Drawing for the job (mm, zero at the part's lowest x, y, z). A direction names the side the tool comes from. Round coordinates to 2 decimals unless told otherwise and drop trailing zeros. Loops run counter-clockwise (first coordinate to the right, second up) from the corner with the lowest first, then second, coordinate; pieces in that order, holes last. Notation, with made-up numbers: M 88,64 L 92,64 A23 ccw 92,73 Z; hole C 82,39.25 d1. An arc over 180 degrees is marked long. Answer in a Markdown table with one row per item.
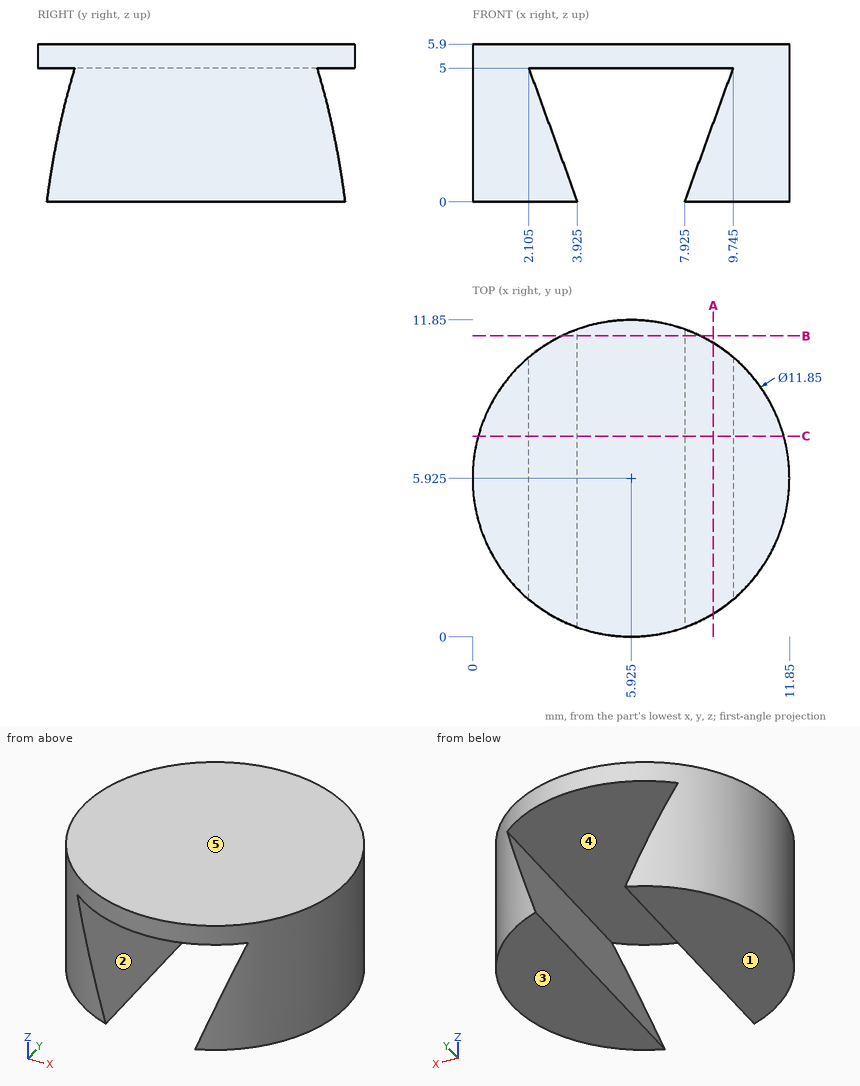
1. Saw through at A-A (x = 9). Write the cut outline in (y, z), and give its area (3 significant figures).
Verdict:
| item | result |
|---|---|
| outline | M 0.86,0 L 10.99,0 L 10.99,2.95 L 0.86,2.95 Z; M 0.86,5 L 10.99,5 L 10.99,5.9 L 0.86,5.9 Z |
| area | 39.0 mm² |
2. Mould opens along Z. For the marked faces 3, 4 and 5 say: +Z half, -Z half, draft (parallel to the pull), parting line (faces both ways), or undercut.
Verdict:
| item | result |
|---|---|
| face 3 | -Z half |
| face 4 | undercut |
| face 5 | +Z half |
3. Tool access for the marked faces 1 and 2: list every direction of +Z, -Z, +X, -X, +Y, -Y with a clear straight run to the whole face (end or side of a thin tool).
Verdict:
| item | result |
|---|---|
| face 1 | -Z, +X, -X, +Y, -Y |
| face 2 | +Y, -Y |
4. Pin check, flat tips, straight feed: pin 1 (4 mm diameter, centred on x = 5, y = 6.5, fed in from -Z); pin 2 (1.5 mm diameter, centred on y = 7.5, z = 5, fed in from -X); pin 3 (2 mm diameter, centred on x = 10.5, z = 2.5, fed in from +Y). Stop position of each tip, or through.
Verdict:
| item | result |
|---|---|
| pin 1 | stops at z = 0 |
| pin 2 | stops at x = 0.06 |
| pin 3 | stops at y = 10.65 |
5. Wall check: probe 1 along X at (y, z) = (5, 0.5); probe 2 along X at (y, z) = (4.25, 1.4) (1 decimal); probe 3 along Z at (x, y) = (5, 10). Give the ranges that are in metal, low to high.
Verdict:
| item | result |
|---|---|
| probe 1 | x = 0.07 to 3.74, 8.11 to 11.78 |
| probe 2 | x = 0.2 to 3.4, 8.4 to 11.6 |
| probe 3 | z = 5 to 5.9 |
6. Saw through at B-B (y = 11.25). Write the cut outline in (x, z) (1 decimal).
Verdict:
| item | result |
|---|---|
| outline | M 3.3,0 L 3.9,0 L 3.3,1.6 Z; M 3.3,5 L 8.5,5 L 8.5,5.9 L 3.3,5.9 Z; M 7.9,0 L 8.5,0 L 8.5,1.6 Z |
7. Saw through at C-C (y = 7.5). Write the cut outline in (x, z) (3 decimals).
Verdict:
| item | result |
|---|---|
| outline | M 0.213,0 L 3.925,0 L 2.105,5 L 9.745,5 L 7.925,0 L 11.637,0 L 11.637,5.9 L 0.213,5.9 Z |
